Design review of the part built by this model. Coordinates are the model's own, in mm. Face numbers are marked on the shaded views. A direction names the side the tool comes from. Coordinates: 2 decimals unless noted, no trailing zeros. Loops run counter-clockwise (first coordinate to the right, second up) from the corner with the lowest first, then second, coordinate; pieces in that order, holes last.
Q1. Machinability: for the marked faces 1 and 2, which of the approach directions +Z, -Z, +X, -X, +Y, -Y give a long, thin tool a straight path to every point of the face, cutting with its end or side? Answer none if there is none.
Q2. For P1, Ø4, axis at x = 10, y = 10, coming from the -Z side; P2, Ø12, axis at x = 12, z = -10.5, coming from the +Y side, all flat-tipped, find the tip position at first contact; note any pin that passes through.
Q3. Wall thickness on probe 1 along X at (y, z) = (-1.2, -27); probe 2 along X at (y, z) = (7.5, -0.35); probe 3 along Z at (x, y) = (4.5, 17.75): over which ranges is each line inside the solid? List them lowest first.
Q4. Add section B-B on x = 10. Give the boundary of the cut face in (y, z), and give its area (3 significant figures).
Q5. Draft analysis for pull direction Z (two halves, no side actions). For the marked faces 3, 4 and 5, state which applies: released by +Z, released by -Z, zero draft, split by the parting line, or undercut.
Q6. Add section D-D on y = 10. Give the boundary of the cut face in (x, z), and give its area (3 significant figures).
Q7. Add section A-A on y = 1.5. Give the boundary of the cut face in (x, z), and give its area (3 significant figures).
Q8. Add section C-C on z = -17. Give the boundary of the cut face in (x, y), and give its area (3 significant figures).
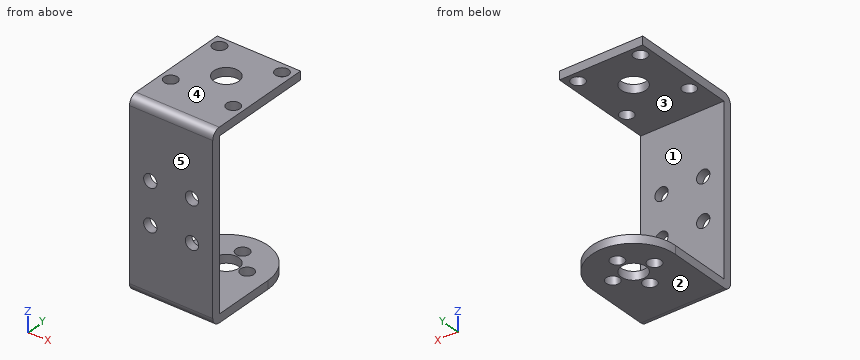
Autodesk Inventor part; units mm, degrees
ref_plane "YZ Plane" through (0, 0, 0) normal (1, 0, 0) x (0, 1, 0)
ref_plane "XZ Plane" through (0, 0, 0) normal (0, 1, 0) x (-1, 0, 0)
ref_plane "XY Plane" through (0, 0, 0) normal (0, 0, 1) x (1, 0, 0)
sketch "スケッチ1" plane through (0, 0, 0) normal (1, 0, 0) x (0, 1, 0)
  line L0 (0, 0) -> (-2, 0)
  line L1 (-2, 0) -> (-2, -44)
  line L2 (-2, -44) -> (0, -44)
  line L3 (0, -44) -> (0, 0)
  line L4 (0, -44) -> (25, -44)
  line L5 (25, -44) -> (25, -42)
  line L6 (25, -42) -> (0, -42)
  line L7 (0, -42) -> (0, -44)
  line L8 (0, 0) -> (25, 0)
  line L9 (25, 0) -> (25, -2)
  line L10 (25, -2) -> (0, -2)
  line L11 (0, -2) -> (0, 0)
  dimension "d0" = 2
  dimension "d1" = 44
  dimension "d2" = 25
  dimension "d3" = 2
  dimension "d4" = 25
  dimension "d5" = 2
extrude "押し出し1" add sketch "スケッチ1" along normal blind 20
sketch "スケッチ2" plane through (0, -2, 0) normal (0, 0, 1) x (1, 0, 0)
  line L0 (0, 27) -> (0, 0)
  line L1 (0, 27) -> (20, 27)
  point P0 (0, 2)
  point P1 (2.5, 24.5)
  point P2 (17.5, 24.5)
  point P3 (17.5, 9.5)
  point P4 (2.5, 9.5)
  dimension "d8" = 2.5
  dimension "d9" = 15
  dimension "d10" = 15
  dimension "d11" = 17.5
hole "穴1" at (2.5, 22.5, 0) at (17.5, 22.5, 0) at (17.5, 7.5, 0) at (2.5, 7.5, 0) direction (0, 0, -1) diameter 3.2 depth 2 tip angle 118
sketch "スケッチ3" plane through (0, -2, 0) normal (0, 0, 1) x (1, 0, 0)
  circle A0 centre (10, 17) radius 3
  line L0 (0, 27) -> (20, 27)
  line L1 (0, 27) -> (0, 0)
  point P0 (0, 2)
  dimension "d19" = 6
  dimension "d20" = 10
  dimension "d21" = 10
extrude "押し出し2" cut sketch "スケッチ3" against normal through all
sketch "スケッチ4" plane through (0, -2, -44) normal (0, 0, -1) x (-1, 0, 0)
  circle A0 centre (-10, 17) radius 3
  circle A1 centre (-10, 17) radius 5
  point P0 (0, 2)
  point P1 (-10, 22)
  point P2 (-15, 17)
  point P3 (-5, 17)
  point P4 (-10, 12)
  dimension "d24" = 10
hole "穴2" at (10, 20, -44) at (15, 15, -44) at (5, 15, -44) at (10, 10, -44) direction (0, 0, 1) diameter 3.2 depth 2 tip angle 118
sketch "スケッチ5" plane through (0, -2, -44) normal (0, 0, -1) x (-1, 0, 0)
  circle A0 centre (-10, 17) radius 3
  circle A1 centre (-10, 17) radius 10
  line L0 (-20, 27) -> (-20, 2)
  line L1 (-20, 17) -> (0, 17)
  line L2 (0, 17) -> (0, 27)
  line L3 (0, 27) -> (-20, 27)
  line L4 (-20, 27) -> (-20, 17)
  point P0 (0, 2)
  point P1 (-10, 27)
  dimension "d32" = 20
extrude "押し出し3" cut sketch "スケッチ5" against normal blind 2 contours A1 L3 L2 | L0 L3 A1
sketch "スケッチ6" plane through (0, -2, -44) normal (0, -1, 0) x (1, 0, 0)
  line L0 (11.6, 0) -> (8.4, 0)
  line L1 (10, 0) -> (10, 44)
  line L2 (7, 44) -> (13, 44)
  line L3 (0, 2) -> (0, 42)
  line L4 (0, 22) -> (20, 22)
  line L5 (20, 2) -> (20, 42)
  point P0 (0, 44)
  point P1 (5, 17)
  point P2 (5, 27)
  point P3 (15, 27)
  point P4 (15, 17)
  dimension "d35" = 10
  dimension "d36" = 10
hole "穴3" at (5, -2, -27) at (5, -2, -17) at (15, -2, -17) at (15, -2, -27) direction (0, 1, 0) diameter 3.2 depth 2 tip angle 118
fillet "フィレット1" radius 2 2 edges at (10, -2, -44) (10, -2, 0)
properties part number "サーボモーター25kgcmサーボホーン3" material "アルミニウム 6061"
Entries:
1. face 1: +X, -X, +Y
1. face 2: -Z, +X, -X, +Y, -Y
2. P1: stops at z = -44
2. P2: stops at y = 0
3. probe 1: x = 0 to 3.4, 6.6 to 13.4, 16.6 to 20
3. probe 2: x = 0 to 0.9, 4.1 to 15.9, 19.1 to 20
3. probe 3: z = -44 to -42, -2 to 0
4. outline: (-2, -42) arc R2 ccw to (0, -44) - (8.4, -44) - (8.4, -42) - (0, -42) - (0, -2) - (12, -2) - (12, 0) - (0, 0) arc R2 ccw to (-2, -2) - close; (11.6, -44) - (12, -44) - (12, -42) - (11.6, -42) - close; (18, -44) - (18.4, -44) - (18.4, -42) - (18, -42) - close; (18, -2) - (25, -2) - (25, 0) - (18, 0) - close; (21.6, -44) - (25, -44) - (25, -42) - (21.6, -42) - close
4. area: 149 mm2
5. face 3: undercut
5. face 4: released by +Z
5. face 5: zero draft
6. outline: (0, -44) - (8.4, -44) - (8.4, -42) - (0, -42) - close; (0, -2) - (20, -2) - (20, 0) - (0, 0) - close; (11.6, -44) - (20, -44) - (20, -42) - (11.6, -42) - close
6. area: 73.6 mm2
7. outline: (0, -44) - (20, -44) - (20, -42) - (0, -42) - close; (0, -2) - (20, -2) - (20, 0) - (0, 0) - close
7. area: 80.0 mm2
8. outline: (0, -2) - (3.4, -2) - (3.4, 0) - (0, 0) - close; (6.6, -2) - (13.4, -2) - (13.4, 0) - (6.6, 0) - close; (16.6, -2) - (20, -2) - (20, 0) - (16.6, 0) - close
8. area: 27.2 mm2
